Can you work these out from the drawing? Everything is in mm from the part's minimum corner. A direction names the side the tool comes from. Give positions to 0.01 mm unless a question says otherwise; leave off trailing zeros. Loops run counter-clockwise (first coordinate to the right, second up) from the corner with the lowest first, then second, coordinate; pieces in that order, holes last. Notation, with made-up numbers: (69, 59.5) -> (115, 59.5) arc R24 cw to (115, 88.5) -> close; hole circle Ø2 at (53.5, 71). An arc over 180 degrees is marked (long way). Return JSON: item names as keys, results as strings. Group by question number.
Q1. Suppose I cut it at D-D, the plane y = 12.5. Please give me the cut outline in (x, z), and give its area (3 significant figures).
Q2. Suppose I cut it at A-A, the plane y = 31.55. Please give me the cut outline in (x, z).
Q3. I need wall thicknesses on line 1 along Z through (x, y) = (47, 10); line 2 along X through (y, z) = (14, 34); line 3 along Z through (x, y) = (27.5, 1.15) (3 decimals). Which ranges of each line are inside material? Lowest first, please. Write a range as [from, to].
Q4. Will these pins go through, and if not, where does the flat tip stop? pin 1 (4.5 mm diameter, centred on y = 29, z = 1.5, fed in from -X); pin 2 (12 mm diameter, centred on x = 46, z = 13, fed in from +Y); pin 3 (13 mm diameter, centred on x = 49.5, y = 9.5, fed in from +Z); pin 4 (2.5 mm diameter, centred on x = 47.5, z = 11.525, fed in from -Y).
Q5. Thinking about a two-plate mould opening in Z: for the marked faces 6, 7 and 8, which applies, pulls with the +Z half, pulls with the -Z half, needs draft (parallel to the pull), parting line crosses it, or undercut?
Q6. Suppose I cut it at C-C, the plane z = 31.6. Please give me the cut outline in (x, y) (3 decimals), and give its area (3 significant figures).
Q7. Which directions (+Z, -Z, +X, -X, +Y, -Y) give clear straight access to the entire face, cutting with the end or side of a thin tool? Please do the marked faces 1, 2, 3, 4 and 5.
Q8. Suppose I cut it at B-B, the plane x = 27.5. Please give me the cut outline in (y, z) (3 decimals).
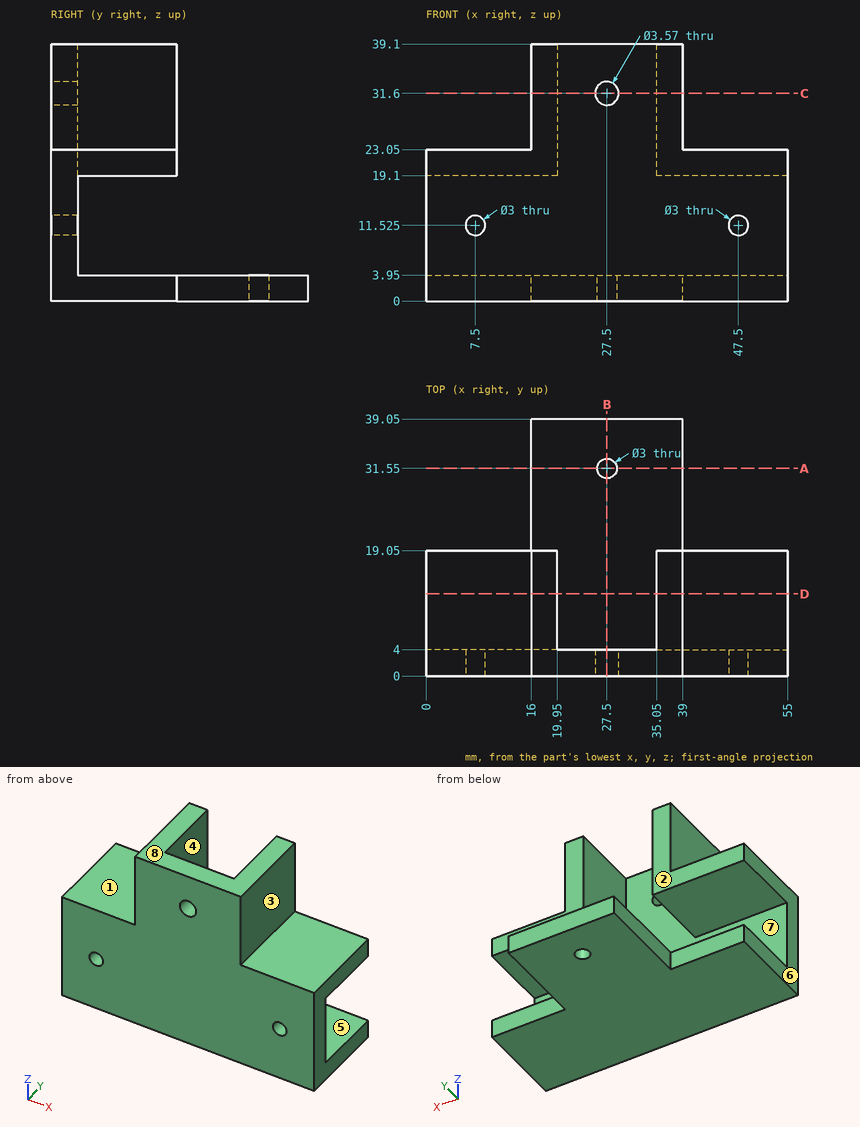
Ans:
{
 "1": {"outline": "(0, 0) -> (55, 0) -> (55, 3.95) -> (0, 3.95) -> close; (0, 19.1) -> (19.95, 19.1) -> (19.95, 39.1) -> (16, 39.1) -> (16, 23.05) -> (0, 23.05) -> close; (35.05, 19.1) -> (55, 19.1) -> (55, 23.05) -> (39, 23.05) -> (39, 39.1) -> (35.05, 39.1) -> close", "area": "502 mm^2"},
 "2": {"outline": "(16, 0) -> (26, 0) -> (26, 3.95) -> (16, 3.95) -> close; (29, 0) -> (39, 0) -> (39, 3.95) -> (29, 3.95) -> close"},
 "3": {"line 1": "z = [0, 3.95], [19.1, 23.05]", "line 2": "x = [16, 19.95], [35.05, 39]", "line 3": "z = [0, 29.815], [33.385, 39.1]"},
 "4": {"pin 1": "stops at x = 16", "pin 2": "stops at y = 4", "pin 3": "stops at z = 23.05", "pin 4": "passes through"},
 "5": {"face 6": "needs draft", "face 7": "undercut", "face 8": "pulls with the +Z half"},
 "6": {"outline": "(16, 0) -> (25.715, 0) -> (25.715, 4) -> (19.95, 4) -> (19.95, 19.05) -> (16, 19.05) -> close; (29.285, 0) -> (39, 0) -> (39, 19.05) -> (35.05, 19.05) -> (35.05, 4) -> (29.285, 4) -> close", "area": "197 mm^2"},
 "7": {"face 1": "+Z, -X, +Y, -Y", "face 2": "+Z, +X, -X, +Y", "face 3": "+Z, +X, +Y, -Y", "face 4": "+Z, +Y", "face 5": "+X, -X, +Y"},
 "8": {"outline": "(0, 0) -> (30.05, 0) -> (30.05, 3.95) -> (4, 3.95) -> (4, 29.815) -> (0, 29.815) -> close; (0, 33.385) -> (4, 33.385) -> (4, 39.1) -> (0, 39.1) -> close; (33.05, 0) -> (39.05, 0) -> (39.05, 3.95) -> (33.05, 3.95) -> close"}
}
